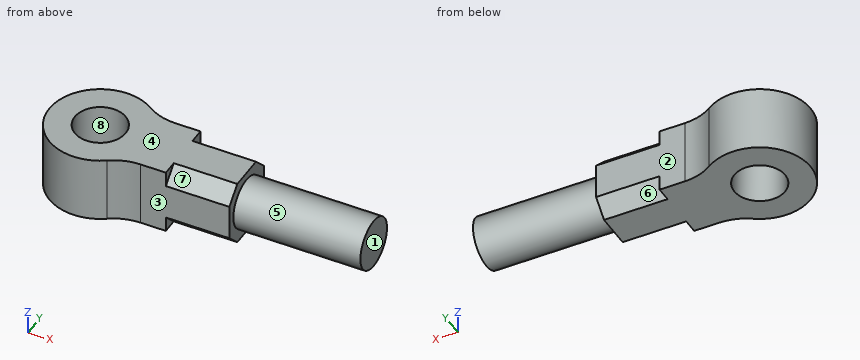
from build123d import *

# Parameters (mm, degrees)
SKETCH1_R           = 10
BOSS_EXTRUDE1_DEPTH = 13
CUT_EXTRUDE1_DEPTH  = 25
SKETCH3_3_R         = 10
BOSS_EXTRUDE2_DEPTH = 50


with BuildPart() as part:
    # Sketch1 → Boss-Extrude1 (new body, symmetric)
    with BuildSketch(Plane.XY):
        with BuildLine():
            Line((57.605309111, 13), (57.605309111, -13))
            Line((57.605309111, -13), (22.605309111, -13))
            ThreePointArc((22.605309111, -13), (16.689229328, -13.895026825), (11.302654555, -16.5))
            ThreePointArc((11.302654555, -16.5), (-20, 0), (11.302654555, 16.5))
            ThreePointArc((11.302654555, 16.5), (16.689229328, 13.895026825), (22.605309111, 13))
            Line((22.605309111, 13), (57.605309111, 13))
        make_face()
        Circle(SKETCH1_R, mode=Mode.SUBTRACT)
    extrude(amount=BOSS_EXTRUDE1_DEPTH, both=True)

    # Sketch3 → Cut-Extrude1 (cut)
    with BuildSketch(Plane(origin=(57.605309111, 0, 0), x_dir=(0, 0, -1), z_dir=(1, 0, 0))):
        Polygon((13, 7), (13, 13), (7, 13), align=None)
        Polygon((13, -13), (13, -7), (7, -13), align=None)
        Polygon((-13, -13), (-7, -13), (-13, -7), align=None)
        Polygon((-13, 13), (-13, 7), (-7, 13), align=None)
    extrude(amount=-CUT_EXTRUDE1_DEPTH, mode=Mode.SUBTRACT)

    # Sketch3_3 → Boss-Extrude2 (add)
    with BuildSketch(Plane(origin=(57.605309111, 0, 0), x_dir=(0, 0, -1), z_dir=(1, 0, 0))):
        Circle(SKETCH3_3_R)
    extrude(amount=BOSS_EXTRUDE2_DEPTH)


solid = part.part
Input: part model. Units: mm. Frame: model coordinates. Face numbers are marked on the shaded views. A direction names the side the tool comes from. Coordinates: 2 decimals unless noted, no trailing zeros. Loops run counter-clockwise (first coordinate to the right, second up) from the corner with the lowest first, then second, coordinate; pieces in that order, holes last. Notation, with made-up numbers: (83, 81.5) -> (114, 81.5) arc R18 ccw to (114, 110.5) -> close; hole circle Ø10 at (62.25, -10.75). An arc over 180 degrees is marked (long way). Write item = value, one per line. Start each with the question number.
Item 1: Cut plane D-D, the plane x = 42. Return loops of the section in (y, z), plus the area to 3 significant figures.
Item 2: Cut plane C-C, the plane z = 0. Return loops of the section in (x, y).
Item 3: Reachability of the marked faces 1, 2, 3, 4 and 5 from +Z, -Z, +X, -X, +Y, -Y: full face, straight path, thin tool, end or side. Return the list, or none.
Item 4: First-contact query: P1, Ø6.5, axis at y = -10.5, z = 8.5, coming from the +X side; P2, Ø5, axis at x = 89, z = 1.5, coming from the +Y side; P3, Ø8, axis at x = 42.5, z = -1, coming from the +Y side. Flat tips, straight axial feed; report the tip coordinate or a pass-through.
Item 5: Cut plane A-A, the plane y = 0. Return loops of the section in (x, z).
Item 6: Mould query, pull axis Y, two halves, no side actions, for the marked faces 6, 7 and 8. Classes: pulls with the +Y half, pulls with the -Y half, needs draft (parallel to the pull), parting line crosses it, or undercut.
Item 7: Cut plane B-B, the plane x = 0. Return loops of the section in (y, z), plus the area to 3 significant figures.
Item 8: Material intervals for line 1 (Y direction, x = 0, z = 2.25); line 2 (Y direction, x = 30, z = 1.75); line 3 (X direction, y = -1.5, z = 2), sorted ascending.
Ans:
q1.outline = (-13, -7) -> (-7, -13) -> (7, -13) -> (13, -7) -> (13, 7) -> (7, 13) -> (-7, 13) -> (-13, 7) -> close
q1.area = 604 mm²
q2.outline = (11.3, -16.5) arc R20 cw to (22.61, -13) -> (57.61, -13) -> (57.61, -10) -> (107.61, -10) -> (107.61, 10) -> (57.61, 10) -> (57.61, 13) -> (22.61, 13) arc R20 cw to (11.3, 16.5) arc R20 ccw (long way) to start; hole circle Ø20 at (0, 0)
q3.face_1 = +Z, -Z, +X, +Y, -Y
q3.face_2 = +Z, -Z, +X, +Y
q3.face_3 = +Z, -Z, +X, -Y
q3.face_4 = +Z, +X, -X, +Y, -Y
q3.face_5 = +X
q4.P1 = 57.61
q4.P2 = 10
q4.P3 = 13
q5.outline = (-20, -13) -> (-10, -13) -> (-10, 13) -> (-20, 13) -> close; (10, -13) -> (57.61, -13) -> (57.61, -10) -> (107.61, -10) -> (107.61, 10) -> (57.61, 10) -> (57.61, 13) -> (10, 13) -> close
q6.face_6 = pulls with the +Y half
q6.face_7 = pulls with the -Y half
q6.face_8 = undercut
q7.outline = (-20, -13) -> (-10, -13) -> (-10, 13) -> (-20, 13) -> close; (10, -13) -> (20, -13) -> (20, 13) -> (10, 13) -> close
q7.area = 520 mm²
q8.line_1 = -20 to -10, 10 to 20
q8.line_2 = -13 to 13
q8.line_3 = -19.94 to -9.89, 9.89 to 107.61
